For this review, take the finished solid that the model builds, in its own axes (mm). A direction names the side the tool comes from. Coordinates: 2 decimals unless noted, no trailing zeros. Write each loop counter-clockwise with the first axis right and the second up, starting at its lowest first coordinate (ties: lowest second). Pieces come first, ordered by that corner, then holes. Notation, with made-up numbers: (40.5, 80) -> (68.5, 80) arc R15 cw to (68.5, 89) -> close; hole circle Ø5 at (85, 19). An arc over 180 degrees is marked (long way). Put each result on its own line as item: value. Start each with the question number.
Item 1: Consider section B-B on y = -6.25. Give the boundary of the cut face in (x, z), and give its area (3 significant figures).
Item 2: For faces 4 (the flat face through (-5.4, -5.1, 2.5)), 5 (the flat face through (5.208, -5.173, 2.514)), 6 (the flat face through (-1, -2, 0)), 7 (the flat face through (5, -1, 2)), list the 3-axis set-ups (+Z, -Z, +X, -X, +Y, -Y) from which the entire face can be reached by the end or side of a thin tool; tool diameter is ignored.
Item 3: Insertion check: P1, Ø1.1, axis at x = -2, y = -5.5, coming from the -Z side; P2, Ø2, axis at x = 3, y = 0.5, coming from the -Z side; P3, Ø1.2, axis at x = 5.5, y = -5.5, coming from the -Z side. Each pin has a flat end and moves straight along its axis. Give the tip position at first contact, or say it passes through.
Item 4: Consider section C-C on x = -2.25. Give the boundary of the cut face in (y, z).
Item 5: The part is to be moulded in two halves that separate along X. For faces 1 (the flat face through (-5.208, -5.173, 2.514)), 2 (the flat face through (-5, -1, 2)), 3 (the flat face through (0, -1, 3.5)), say which applies: +X half, -X half, draft (parallel to the pull), parting line (faces both ways), or undercut.
Item 6: To check wall thickness, follow L1, parallel to X at y = -3.5, z = 3.3; L2, parallel to Y at x = -0.5, z = 2.85; L3, parallel to X at y = -5, z = 2.55. State the ranges of each line that lie inside material, in increasing order.
Item 7: Consider section D-D on y = -3.25. Give the boundary of the cut face in (x, z).
```python
from build123d import *

# Parameters (mm, degrees)
BOSS_EXTRU_1_DEPTH             = 3.5
ESQUISSE2_R                    = 1.75
BOSS_EXTRU_2_DEPTH             = 0.5
CONG_1_R                       = 0.25
BOSS_EXTRU_3_START             = -0.1
BOSS_EXTRU_3_DEPTH             = 0.15
R_P_TITION_LIN_AIRE1_COUNT     = 2
R_P_TITION_LIN_AIRE1_PITCH     = 2
R_P_TITION_LIN_AIRE1_COL_COUNT = 2
R_P_TITION_LIN_AIRE1_COL_PITCH = 2
CHANFREIN1_SIZE                = 1
EXTRU_MINCE1_DEPTH             = 2
CONG_2_R                       = 0.75
CONG_3_R                       = 0.75


with BuildPart() as part:
    # Esquisse1 → Boss.-Extru.1 (new body)
    with BuildSketch(Plane.XY):
        with BuildLine():
            Line((-5, 2.5), (-5, -4.5))
            Line((-5, -4.5), (5, -4.5))
            Line((5, -4.5), (5, 2.5))
            ThreePointArc((5, 2.5), (2.692582404, 3.981456009), (0, 4.5))
            ThreePointArc((0, 4.5), (-2.692582404, 3.981456009), (-5, 2.5))
        make_face()
        Polygon((-0.288675135, 0.5), (-0.577350269, 0), (-0.288675135, -0.5), (0.288675135, -0.5), (0.577350269, 0), (0.288675135, 0.5), align=None, mode=Mode.SUBTRACT)
    extrude(amount=BOSS_EXTRU_1_DEPTH)

    # Esquisse2 → Boss.-Extru.2 (add)
    with BuildSketch(Plane.XY):
        Circle(ESQUISSE2_R)
        Polygon((-0.577350269, 0), (-0.288675135, -0.5), (0.288675135, -0.5), (0.577350269, 0), (0.288675135, 0.5), (-0.288675135, 0.5), align=None, mode=Mode.SUBTRACT)
    extrude(amount=-BOSS_EXTRU_2_DEPTH)

    # Congé1
    cong_1_edges = [part.edges().sort_by_distance(p)[0] for p in [
        (-1.75, 0, 0),
    ]]
    fillet(cong_1_edges, radius=CONG_1_R)

    # Esquisse3 → Boss.-Extru.3 (add)
    with BuildSketch(Plane.XY.offset(3.5).offset(BOSS_EXTRU_3_START)):
        with BuildLine():
            Line((-0.5, -4.5), (-0.5, -7.5))
            ThreePointArc((-0.5, -7.5), (0, -8), (0.5, -7.5))
            Line((0.5, -7.5), (0.5, -4.5))
            Line((0.5, -4.5), (-0.5, -4.5))
        make_face()
    boss_extru_3 = extrude(amount=-BOSS_EXTRU_3_DEPTH)

    # Répétition linéaire1: Boss.-Extru.3 ×2
    with Locations(*[(i * R_P_TITION_LIN_AIRE1_PITCH, 0, 0) for i in range(1, R_P_TITION_LIN_AIRE1_COUNT)]):
        add(boss_extru_3)

    # Répétition linéaire1 col: Boss.-Extru.3 ×2
    with Locations(*[(-i * R_P_TITION_LIN_AIRE1_COL_PITCH, 0, 0) for i in range(1, R_P_TITION_LIN_AIRE1_COL_COUNT)]):
        add(boss_extru_3)

    # Chanfrein1
    chanfrein1_edges = [part.edges().sort_by_distance(p)[0] for p in [
        (5, -4.5, 1.75),
        (-5, -4.5, 1.75),
    ]]
    chamfer(chanfrein1_edges, length=CHANFREIN1_SIZE)

    # Esquisse4 → Extru.-Mince1 (add)
    with BuildSketch(Plane.XY.offset(3.5)):
        Polygon((-5, -3.5), (-5, -4.5), (-6, -6), (-5, -7.5), (-4.833589941, -7.389059961), (-5.759629915, -6), (-4.8, -4.560555128), (-4.8, -3.5), align=None)
    extru_mince1 = extrude(amount=-EXTRU_MINCE1_DEPTH)

    # Symétrie1: Extru.-Mince1 across plane
    add(extru_mince1.mirror(Plane.ZY))

    # Congé2
    cong_2_edges = [part.edges().sort_by_distance(p)[0] for p in [
        (-4.916794971, -7.44452998, 3.5),
        (-4.916794971, -7.44452998, 1.5),
        (4.916794971, -7.44452998, 1.5),
        (4.916794971, -7.44452998, 3.5),
    ]]
    fillet(cong_2_edges, radius=CONG_2_R)

    # Congé3
    cong_3_edges = [part.edges().sort_by_distance(p)[0] for p in [
        (-6, -6, 2.5),
        (-5, -4.5, 2.5),
        (-4.8, -4.560555128, 2.5),
        (-5.759629915, -6, 2.5),
        (6, -6, 2.5),
        (5.759629915, -6, 2.5),
        (4.8, -4.560555128, 2.5),
        (5, -4.5, 2.5),
    ]]
    fillet(cong_3_edges, radius=CONG_3_R)


solid = part.part
```
Return value:
1. outline: (-5.81, 1.5) -> (-5.57, 1.5) -> (-5.57, 3.5) -> (-5.81, 3.5) -> close; (-2.5, 3.25) -> (-1.5, 3.25) -> (-1.5, 3.4) -> (-2.5, 3.4) -> close; (-0.5, 3.25) -> (0.5, 3.25) -> (0.5, 3.4) -> (-0.5, 3.4) -> close; (1.5, 3.25) -> (2.5, 3.25) -> (2.5, 3.4) -> (1.5, 3.4) -> close; (5.57, 1.5) -> (5.81, 1.5) -> (5.81, 3.5) -> (5.57, 3.5) -> close
1. area: 1.41 mm^2
2. face 4: +Z, -Z, -X, +Y
2. face 5: +Z, -Z
2. face 6: -Z
2. face 7: +Z, -Z, +X, +Y
3. P1: z = 3.25
3. P2: z = 0
3. P3: z = 1.5
4. outline: (-7.93, 3.25) -> (-4.5, 3.25) -> (-4.5, 0) -> (4.14, 0) -> (4.14, 3.5) -> (-4.5, 3.5) -> (-4.5, 3.4) -> (-7.93, 3.4) -> close
5. face 1: undercut
5. face 2: -X half
5. face 3: draft
6. L1: -5 to 5
6. L2: -4.5 to -0.13, 0.13 to 4.48
6. L3: -5.33 to -5.09, 5.09 to 5.33
7. outline: (-5, 0) -> (5, 0) -> (5, 3.5) -> (-5, 3.5) -> close
